from build123d import *

# Parameters (mm, degrees)
SKETCH1_R           = 7.5
BOSS_EXTRUDE1_DEPTH = 12
SKETCH2_R           = 15
BOSS_EXTRUDE2_DEPTH = 180


with BuildPart() as part:
    # Sketch1 → Boss-Extrude1 (new body)
    with BuildSketch(Plane(origin=(0, 0, 0), x_dir=(1, 0, 0), z_dir=(0, 1, 0))):
        with BuildLine():
            Line((0, 15), (35, 15))
            ThreePointArc((35, 15), (50, 0), (35, -15))
            Line((35, -15), (0, -15))
            ThreePointArc((0, -15), (-15, 0), (0, 15))
        make_face()
        with Locations(Location((35, 0, 0), (0, 0, 270))):  # turned: the seam where the file's is
            Circle(SKETCH1_R, mode=Mode.SUBTRACT)
    extrude(amount=BOSS_EXTRUDE1_DEPTH)

    # Sketch2 → Boss-Extrude2 (add)
    with BuildSketch(Plane(origin=(0, 12, 0), x_dir=(1, 0, 0), z_dir=(0, 1, 0))):
        with Locations(Location((0, 0, 0), (0, 0, 270))):  # turned: the seam where the file's is
            Circle(SKETCH2_R)
    extrude(amount=BOSS_EXTRUDE2_DEPTH)

    # Sketch3 → Revolve1 (revolve)
    with BuildSketch(Plane(origin=(0, 0, 0), x_dir=(0, 0, -1), z_dir=(1, 0, 0)), mode=Mode.PRIVATE) as revolve1_sk:
        Polygon((15, 192), (0, 192), (0, 217.980762114), align=None)
    revolve(revolve1_sk.sketch.rotate(Axis((0, -19.330259434, 0), (0, 1, 0)), 180), axis=Axis((0, -19.330259434, 0), (0, 1, 0)))  # turned: the seam where the file's is


solid = part.part
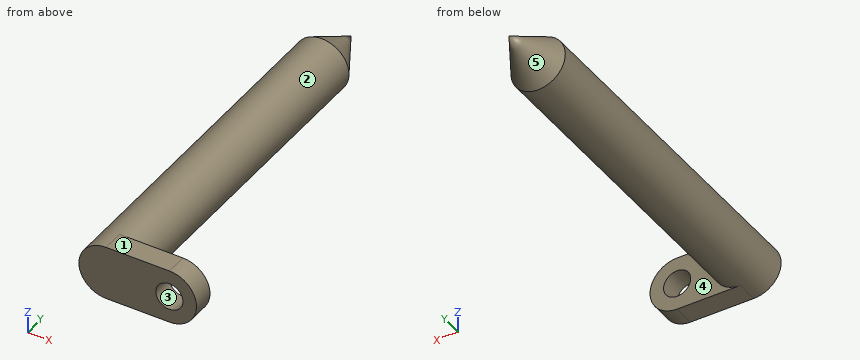
Part model, mm, in its own coordinate system. Face numbers are marked on the shaded views. A direction names the side the tool comes from. Coordinates: 2 decimals unless noted, no trailing zeros. Loops run counter-clockwise (first coordinate to the right, second up) from the corner with the lowest first, then second, coordinate; pieces in that order, holes last. Notation, with made-up numbers: (60, 77) -> (93, 77) arc R22 cw to (93, 99) -> close; hole circle Ø7 at (43.25, 55.25). An arc over 180 degrees is marked (long way). Use a Markdown table: item, result. Add a question column.
Item 1: Probe probe 1 along X at (y, z) = (4.75, 0); probe 2 along Y at (x, z) = (44.5, -2.5); probe 3 along X at (y, z) = (70, -13). List the from-to ranges inside material, lowest first.
Item 2: Band-saw the part on B-B on y = 130. Write the cut outline in (x, z), plus the area to 3 significant figures.
Item 3: Band-saw the part on A-A on x = 21. Write the cut outline in (y, z), plus the area to 3 significant figures.
Item 4: Flat gauge pins, fed straight in: P1, Ø3, axis at x = 11, y = 77, coming from the -Z side; P2, Ø10, axis at y = 99, z = 0.5, coming from the -X side; P3, Ø6, axis at x = -7, y = 124, coming from the -Z side; P4, Ø10, axis at y = 164, z = -6.5, coming from the +X side. Where does each tip first touch, or does it go through?
Item 5: Which spindle directions (+Z, -Z, +X, -X, +Y, -Y) get a long thin tool onto all of the face, cutting with end or side? Do the marked faces 1 and 2. Say none if no direction does.
Item 6: Pull direction Z, two halves, no side cores. Call the marked faces 3, 4 and 5: +Z half, -Z half, draft (parallel to the pull), parting line (faces both ways), or undercut.
Geometry says:
| question | item | result |
|---|---|---|
| 1 | probe 1 | -15 to 27.5, 42.5 to 50 |
| 1 | probe 2 | 0 to 12 |
| 1 | probe 3 | -7.48 to 7.48 |
| 2 | outline | circle Ø30 at (0, 0) |
| 2 | area | 707 mm² |
| 3 | outline | (0, -15) -> (12, -15) -> (12, 15) -> (0, 15) -> close |
| 3 | area | 360 mm² |
| 4 | P1 | z = -11.61 |
| 4 | P2 | x = -15 |
| 4 | P3 | z = -14.46 |
| 4 | P4 | x = 14.92 |
| 5 | face 1 | +Z, +X, -X, +Y, -Y |
| 5 | face 2 | +Y |
| 6 | face 3 | undercut |
| 6 | face 4 | draft |
| 6 | face 5 | parting line |
